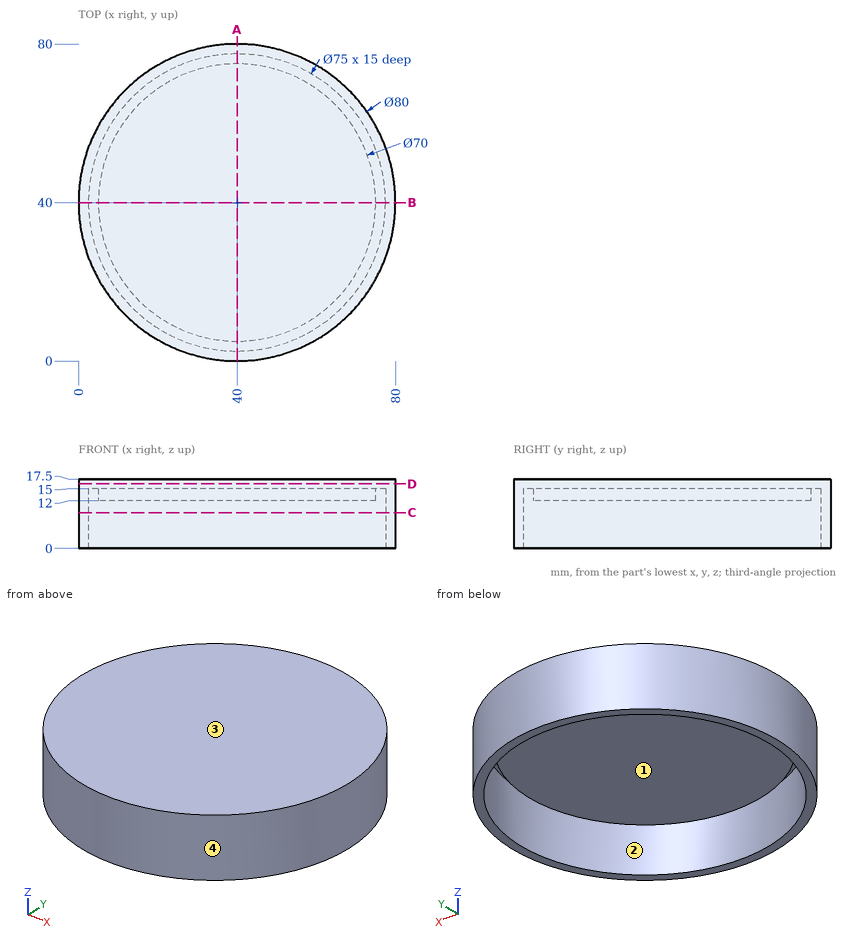
Geometry: see drawing. Coordinates: mm, zero at the bounding-box minimum. Give positions to 0.01 mm unless a question says otherwise; leave off trailing zeros. Write each loop counter-clockwise with the first axis right and the second up, starting at its lowest first coordinate (ties: lowest second). Pieces come first, ordered by that corner, then holes. Notation, with made-up numbers: (54.25, -22) - (101.25, -22) arc R18 ccw to (101.25, 4) - close; hole circle Ø10 at (67, 45). An arc over 180 degrees is marked (long way). Return JSON: item names as keys, results as strings. Group by question number.
1) Section C-C on z = 9. Return the cut outline in (x, y), plus the area to 3 significant figures.
2) First-contact query: P1, Ø1.5, axis at x = 25, z = 2, coming from the +Y side; P2, Ø6, axis at x = 63.5, z = 10, coming from the -Y side; P3, Ø6, axis at x = 51, z = 7, coming from the -Y side. Flat tips, straight axial feed; report the tip coordinate or a pass-through.
3) Section D-D on z = 16.25. Return the cut outline in (x, y), plus the area to 3 significant figures.
4) Mould query, pull axis X, two halves, no side actions, for the marked faces 1, 2, 3 and 4. Classes: released by +X, released by -X, zero draft, split by the parting line, or undercut.
5) Line query: line 1 (Y direction, x = 40, z = 8.5); line 2 (X direction, y = 14, z = 13.25); line 3 (Y direction, x = 53.5, z = 14.75). Output: solid intervals per line, ascending.
6) Section A-A on x = 40. Return the cut outline in (y, z), plus the area to 3 significant figures.
Filled in:
{
 "1": {"outline": "circle Ø80 at (40, 40); hole circle Ø75 at (40, 40)", "area": "609 mm^2"},
 "2": {"P1": "stops at y = 77.38", "P2": "stops at y = 5.65", "P3": "stops at y = 0.81"},
 "3": {"outline": "circle Ø80 at (40, 40)", "area": "5,030 mm^2"},
 "4": {"face 1": "undercut", "face 2": "undercut", "face 3": "zero draft", "face 4": "split by the parting line"},
 "5": {"line 1": "y = 0 to 2.5, 77.5 to 80", "line 2": "x = 9.6 to 12.98, 16.57 to 63.43, 67.02 to 70.4", "line 3": "y = 2.35 to 5.01, 7.71 to 72.29, 74.99 to 77.65"},
 "6": {"outline": "(0, 0) - (2.5, 0) - (2.5, 15) - (5, 15) - (5, 12) - (75, 12) - (75, 15) - (77.5, 15) - (77.5, 0) - (80, 0) - (80, 17.5) - (0, 17.5) - close", "area": "485 mm^2"}
}
